For this review, take the finished solid that the model builds, in its own axes (mm). A direction names the side the tool comes from. Coordinates: 2 decimals unless noted, no trailing zeros. Write each loop counter-clockwise with the first axis right and the second up, starting at its lowest first coordinate (ties: lowest second). Pieces come first, ordered by that corner, then holes. Notation, with made-up numbers: M 64,29 L 120,29 A21 ccw 120,55 Z; hole C 46.5,18.5 d11. An arc over 180 degrees is marked long. One line per question, with ' | ' between items.
from build123d import *

# Parameters (mm, degrees)
SKETCH2_R          = 5
CUT_EXTRUDE1_DEPTH = 91.997252706


with BuildPart() as part:
    # Sketch1 → Revolve1 (revolve)
    with BuildSketch(Plane.XY, mode=Mode.PRIVATE) as revolve1_sk:
        Polygon((-45, 0), (45, 0), (45, 9.5), (32.75, 9.5), (32.75, 7.5), (29.45, 7.5), (29.45, 9.5), (17.2, 9.5), (17.2, 7.5), (13.9, 7.5), (13.9, 9.5), (1.65, 9.5), (1.65, 7.5), (-1.65, 7.5), (-1.65, 9.5), (-13.9, 9.5), (-13.9, 7.5), (-17.2, 7.5), (-17.2, 9.5), (-29.45, 9.5), (-29.45, 7.5), (-32.75, 7.5), (-32.75, 9.5), (-45, 9.5), align=None)
    revolve(revolve1_sk.sketch.rotate(Axis((-45, 0, 0), (1, 0, 0)), 180), axis=Axis((-45, 0, 0), (1, 0, 0)))

    # Sketch2 → Cut-Extrude1 (cut, through all)
    with BuildSketch(Plane(origin=(45, 0, 0), x_dir=(0, 0, -1), z_dir=(1, 0, 0))):
        with Locations(Location((0, 0, 0), (0, 0, 90))):
            Circle(SKETCH2_R)
    extrude(amount=-CUT_EXTRUDE1_DEPTH, mode=Mode.SUBTRACT)


solid = part.part
1. Draft analysis for pull direction X (two halves, no side actions). For faces 3 (the cylindrical face through (-23.411, 2.059, 9.274)), 4 (the flat face through (-29.45, -1, -8)), 5 (the flat face through (45, 4, 4)), state which applies: pulls with the +X half, pulls with the -X half, needs draft (parallel to the pull), parting line crosses it, or undercut.
Computed values:
face 3: needs draft | face 4: undercut | face 5: pulls with the +X half
2. Machinability: for faces 1 (the cylindrical face through (38.789, 2.059, 9.274)), 2 (the flat face through (-32.75, 1, -8)), which of the approach directions +Z, -Z, +X, -X, +Y, -Y give a long, thin tool a straight path to every point of the face, cutting with its end or side? Answer none if there is none.
Computed values:
face 1: +X, -X | face 2: none
3. Clearance check with flat-ended pins moving along their axes: P1, Ø5.5, axis at y = -1.5, z = -1.5, coming from the -X side; P2, Ø6, axis at x = -1.5, z = -2.5, coming from the -Y side; P3, Ø1.5, axis at x = 12.5, y = 2.5, coming from the +Z side; P4, Ø8, axis at x = -11, y = -5, coming from the +Z side. State where each tip first meets the part, or that it passes through.
Computed values:
P1: passes through | P2: stops at y = -9.5 | P3: stops at z = 9.34 | P4: stops at z = 9.45
4. For line 1 along X through (y, z) = (-3.5, -8.5); line 2 along Z through (x, y) = (-14.5, 0); line 3 along Z through (x, y) = (12, 0), list the stretches that pass through material, from the lowest coordinate up.
Computed values:
line 1: x = -45 to -32.75, -29.45 to -17.2, -13.9 to -1.65, 1.65 to 13.9, 17.2 to 29.45, 32.75 to 45 | line 2: z = -7.5 to -5, 5 to 7.5 | line 3: z = -9.5 to -5, 5 to 9.5
5. Take a section at A-A on x = -34. State the section outline as (y, z) points.
Computed values:
outline: C 0,0 d19; hole C 0,0 d10
